Read the model definition and answer for the solid it produces. Units are mm, in the model's axes. Give positions to 0.01 mm unless a question says otherwise; leave off trailing zeros. Write each loop counter-clockwise with the first axis right and the second up, starting at its lowest first coordinate (ties: lowest second). Pieces come first, ordered by that corner, then holes. Notation, with made-up numbers: (24.5, -28) - (68.5, -28) arc R27 cw to (68.5, 10) - close; hole circle Ø7 at (65.5, 34.5). An arc over 180 degrees is marked (long way). Answer as CSV lines item,"result".
Autodesk Inventor part; units mm, degrees
ref_plane "Work Plane1" through (-19.1723, 0, 0) normal (0, -0.866, -0.5) x (1, 0, 0)
ref_plane "YZ Plane" through (0, 0, 0) normal (1, 0, 0) x (0, 1, 0)
ref_plane "XZ Plane" through (0, 0, 0) normal (0, 1, 0) x (-1, 0, 0)
sketch "Эскиз1" plane through (0, 0, 0) normal (1, 0, 0) x (0, 1, 0)
  line L0 (-9.815, 0) -> (-4.9075, 8.5)
  line L1 (-4.9075, 8.5) -> (4.9075, 8.5)
  line L2 (4.9075, 8.5) -> (9.815, 0)
  line L3 (9.815, 0) -> (4.9075, -8.5)
  line L4 (4.9075, -8.5) -> (-4.9075, -8.5)
  line L5 (-4.9075, -8.5) -> (-9.815, 0)
  point P0 (0, 0)
  point P1 (0, 0)
  dimension "d0" = 19.6299
extrude "Базовый элемент" add sketch "Эскиз1" along normal blind 8
sketch "Эскиз2" plane through (0, 0, 0) normal (0, 0, 1) x (1, 0, 0)
  line L0 (0, 4.9075) -> (0, 9.815)
  line L1 (0, 9.815) -> (8, 9.815)
  line L2 (8, 4.9075) -> (8, 9.815)
  line L3 (-1.6, 0) -> (9.6, 0)
  line L4 (0.7592, 9.815) -> (0, 8.5)
  line L5 (7.2408, 9.815) -> (8, 8.5)
  dimension "d3" = 30
  dimension "d4" = 30
  dimension "d5" = 17
  dimension "d6" = 17
revolve "Фаска1" cut sketch "Эскиз2" angle 360 about axis through (-10, 0, 0) along (1, 0, 0)
sketch "Эскиз3" plane through (8, 0, 0) normal (1, 0, 0) x (0, 0, -1)
  arc A0 (-4.25, -7.3612) -> (4.25, -7.3612) centre (0, 0) ccw
hole "Резьба" at (8, 0, 0) direction (-1, 0, 0) diameter 8.376 end through all
chamfer "Фаска2" distance 0.8119 angle 30 1 edges at (8, 0, 4.188) measured on face at (8, 7.0214, -0.1683)
chamfer "Фаска3" distance 0.8119 angle 30 1 edges at (0, 0, 4.188) measured on face at (0, 7.0214, -0.1683)
ref_plane "Work Plane1" through (-19.1723, 0, 0) normal (0, -0.866, -0.5) x (1, 0, 0)
equation "\"d0\" = 1.1547 * SW"
equation "\"d1\" = KOH"
equation "\"d3\" = ANG1"
equation "\"d4\" = ANG2"
equation "\"d5\" = SW0"
equation "\"d6\" = SW01"
equation "\"d8\" = -0.5 * GD1 + 0.5 * NND"
equation "\"d40\" = -0.5 * GD1 + 0.5 * NND"
equation "\"d10\" = -0.5 * GD1 + 0.5 * NND"
equation "\"d41\" = -0.5 * GD1 + 0.5 * NND"
equation "\"ANG1\" = 30deg"
equation "\"ANG2\" = 30deg"
equation "\"KOH\" = 8"
equation "\"SW\" = 17"
equation "\"SW0\" = 17"
equation "\"SW01\" = SW0"
equation "\"GUL\" = 0.541266 * PTC"
equation "\"LADI\" = 16.15"
equation "\"TOA\" = 30deg"
equation "\"FAWI\" = 30deg"
equation "\"PTC\" = 1.5"
equation "\"E0\" = 1.155 * SW"
equation "\"GAL\" = 0.541266 * PTC"
properties part number "Гайка M10-6H ГОСТ 5927-70" material "Сталь, мягкая"
(1) The mould has two halves that part along Z. Classify faces 1 (the flat face through (0, 4, -4)), 2 (the flat face through (4, 0, -8.5)), 3 (the cylindrical face through (3.951, -2.83, 3.087)), 4 (the conical face through (7.87, 8.72, 0.19)): +Z half, -Z half, draft (parallel to the pull), parting line (faces both ways), or undercut.
Worked out:
face 1,"draft"
face 2,"-Z half"
face 3,"undercut"
face 4,"parting line"
(2) A cutting plane is placed at A-A (x = 1.5). Write down the section's boundary in (y, z) (1 decimal).
Worked out:
outline,"(-9.8, 0) - (-4.9, -8.5) - (4.9, -8.5) - (9.8, 0) - (4.9, 8.5) - (-4.9, 8.5) - close; hole circle Ø8.4 at (0, 0)"
(3) Each of these flat-tipped pins is pushed along its axis until it touches: P1, Ø2, axis at x = 1.5, y = 7, coming from the +Z side; P2, Ø2, axis at x = 1.5, z = 6.5, coming from the +Y side; P3, Ø7.5, axis at y = 0, z = 0, coming from the -X side. Where does it stop, or does it pass through?
Worked out:
P1,"stops at z = 6.61"
P2,"stops at y = 6.64"
P3,"passes through"
(4) Find the intervals of material crossed by L1, parallel to Z at x = 5.75, y = 0; L2, parallel to Y at x = 5, z = 0.75; L3, parallel to Y at x = 5.5, z = -3.25, in increasing order.
Worked out:
L1,"z = -8.5 to -4.19, 4.19 to 8.5"
L2,"y = -9.38 to -4.12, 4.12 to 9.38"
L3,"y = -7.94 to -2.64, 2.64 to 7.94"
